Solid Edge part; units mm, degrees
sketch "Sketch1" plane through (0, 0, 0) normal (-1, 0, 0) x (0, -1, 0)
  line L0 (-34.86, -50.21) -> (34.86, -50.21)
  line L1 (34.86, -50.21) -> (34.86, 50.21)
  line L2 (34.86, 50.21) -> (-34.86, 50.21)
  line L3 (-34.86, 50.21) -> (-34.86, -50.21)
extrude "Protrusion1" add sketch "Sketch1" along normal blind 6.67
sketch "Sketch2" plane through (-6.67, 0, 0) normal (-1, 0, 0) x (0, -1, 0)
  circle A0 centre (-32.16, 36.8) radius 1.5
  circle A1 centre (32.16, 36.8) radius 1.5
  circle A2 centre (-32.16, -41.22) radius 1.5
  circle A3 centre (32.16, -41.22) radius 1.5
extrude "Cutout1" cut sketch "Sketch2" against normal blind 15
fillet "Round_7" radius 2 4 edges at (-6.67, 0, 50.21) (-6.67, 0, -50.21) (-3.335, 34.86, -50.21) (-3.335, -34.86, -50.21)
Work out the finished part from the listing and answer in its coordinate system (mm). Round coordinates to 2 decimals unless told otherwise and drop trailing zeros. Loops run counter-clockwise (first coordinate to the right, second up) from the corner with the lowest first, then second, coordinate; pieces in that order, holes last. Notation, with made-up numbers: M -18,20.5 L 6,20.5 A13 cw 6,29.5 Z; hole C 44,-33.5 d1. An arc over 180 degrees is marked long. Use CSV: the item, a comma, the result in double quotes.
Q1. Consider L1, parallel to Z at x = -2, y = 32.16; L2, parallel to Z at x = -2.5, y = 31; L3, parallel to Y at x = -5, z = 37.5. Determine where each line is inside the solid, lowest interval first.
Determined:
L1,"-50.21 to -42.72, -39.72 to 35.3, 38.3 to 50.21"
L2,"-50.21 to -42.17, -40.27 to 35.85, 37.75 to 50.21"
L3,"-34.86 to -33.49, -30.83 to 30.83, 33.49 to 34.86"
Q2. Section A-A, the plane z = -41.22 is taken. Determine the outline of the cut face in (x, y).
Determined:
outline,"M -6.67,-34.86 L 0,-34.86 L 0,-33.66 L -6.67,-33.66 Z; M -6.67,-30.66 L 0,-30.66 L 0,30.66 L -6.67,30.66 Z; M -6.67,33.66 L 0,33.66 L 0,34.86 L -6.67,34.86 Z"
Q3. The mould has two halves that part along Y. Classify faces 1 (the flat face through (0, 0, 1)), 2 (the cylindrical face through (-3.38, 30.73, -40.77)), 3 (the cylindrical face through (-3.4, 34.3, -49.6)): pulls with the +Y half, pulls with the -Y half, needs draft (parallel to the pull), parting line crosses it, or undercut.
Determined:
face 1,"needs draft"
face 2,"undercut"
face 3,"pulls with the +Y half"
